Here's how the part is built. I have some questions about the finished solid (model axes, mm). Give positions to 0.01 mm unless a question says otherwise; leave off trailing zeros. Order: outer loops, then holes, each group sorted by start corner. A loop starts at its lowest first (then second) coordinate and runs counter-clockwise, first axis right, second up.
from build123d import *

# Parameters (mm, degrees)
BOSS_EXTRUDE4_DEPTH = 200
SKETCH3_R           = 2
CUT_EXTRUDE1_DEPTH  = 200
SKETCH3_3_R         = 3
SKETCH3_3_R_2       = 2
CUT_EXTRUDE2_DEPTH  = 2.5
SKETCH4_W           = 36.815771896
SKETCH4_H           = 9
CUT_EXTRUDE3_DEPTH  = 10


with BuildPart() as part:
    # Sketch1 → Boss-Extrude4 (new body)
    with BuildSketch(Plane.XY):
        with BuildLine():
            Line((10.168613541, -5.014716436), (10.168390302, 3.235283561))
            Line((10.168390302, 3.235283561), (9.793380155, 3.610273413))
            Line((9.793380155, 3.610273413), (7.005880156, 3.610197985))
            Line((7.005880156, 3.610197985), (6.630890303, 3.235187838))
            Line((6.630890303, 3.235187838), (6.630908906, 2.547687839))
            ThreePointArc((6.630908906, 2.547687839), (6.508267883, 2.251583555), (6.212170237, 2.128926508))
            ThreePointArc((6.212170237, 2.128926508), (5.916065954, 2.251567531), (5.793408907, 2.547665177))
            Line((5.793408907, 2.547665177), (5.793390303, 3.235165176))
            Line((5.793390303, 3.235165176), (5.418380156, 3.610155029))
            Line((5.418380156, 3.610155029), (4.793380156, 3.610138117))
            Line((4.793380156, 3.610138117), (4.168397069, 2.985121205))
            Line((4.168397069, 2.985121205), (4.168606778, -4.764878792))
            Line((4.168606778, -4.764878792), (4.79362369, -5.38986188))
            Line((4.79362369, -5.38986188), (5.41862369, -5.389844968))
            Line((5.41862369, -5.389844968), (5.793613542, -5.014834821))
            Line((5.793613542, -5.014834821), (5.793594939, -4.327334821))
            ThreePointArc((5.793594939, -4.327334821), (6.212333608, -3.90857349), (6.631094939, -4.327312159))
            Line((6.631094939, -4.327312159), (6.631113542, -5.014812159))
            Line((6.631113542, -5.014812159), (7.006123689, -5.389802011))
            Line((7.006123689, -5.389802011), (9.793623688, -5.389726583))
            Line((9.793623688, -5.389726583), (10.168613541, -5.014716436))
        make_face()
    extrude(amount=BOSS_EXTRUDE4_DEPTH)

    # Sketch3 → Cut-Extrude1 (cut)
    with BuildSketch(Plane(origin=(4.168477841, 0.000112796, 0), x_dir=(0, 0, 1), z_dir=(-0.999999999633898, -2.7059269393071615e-05, 0))):
        with Locations(Location((9, -0.88999159, 0), (0, 0, 270))):
            Circle(SKETCH3_R)
        with Locations(Location((29, -0.88999159, 0), (0, 0, 270))):
            Circle(SKETCH3_R)
        with Locations(Location((49, -0.88999159, 0), (0, 0, 270))):
            Circle(SKETCH3_R)
        with Locations(Location((69, -0.88999159, 0), (0, 0, 270))):
            Circle(SKETCH3_R)
        with Locations(Location((89, -0.88999159, 0), (0, 0, 270))):
            Circle(SKETCH3_R)
        with Locations(Location((109, -0.88999159, 0), (0, 0, 270))):
            Circle(SKETCH3_R)
        with Locations(Location((129, -0.88999159, 0), (0, 0, 270))):
            Circle(SKETCH3_R)
        with Locations(Location((149, -0.88999159, 0), (0, 0, 270))):
            Circle(SKETCH3_R)
        with Locations(Location((169, -0.88999159, 0), (0, 0, 270))):
            Circle(SKETCH3_R)
        with Locations(Location((189, -0.88999159, 0), (0, 0, 270))):
            Circle(SKETCH3_R)
    extrude(amount=-CUT_EXTRUDE1_DEPTH, mode=Mode.SUBTRACT)

    # Sketch3_3 → Cut-Extrude2 (cut)
    # profile 1 of 10: a face of its own
    with BuildSketch(Plane(origin=(4.168477841, 0.000112796, 0), x_dir=(0, 0, 1), z_dir=(-0.999999999633898, -2.7059269393071615e-05, 0))):
        with Locations(Location((9, -0.88999159, 0), (0, 0, 270))):
            Circle(SKETCH3_3_R)
        with Locations(Location((9, -0.88999159, 0), (0, 0, 270))):
            Circle(SKETCH3_3_R_2, mode=Mode.SUBTRACT)
    # profile 2 of 10: a face of its own
    with BuildSketch(Plane(origin=(4.168477841, 0.000112796, 0), x_dir=(0, 0, 1), z_dir=(-0.999999999633898, -2.7059269393071615e-05, 0))):
        with Locations(Location((29, -0.88999159, 0), (0, 0, 270))):
            Circle(SKETCH3_3_R)
        with Locations(Location((29, -0.88999159, 0), (0, 0, 270))):
            Circle(SKETCH3_3_R_2, mode=Mode.SUBTRACT)
    # profile 3 of 10: a face of its own
    with BuildSketch(Plane(origin=(4.168477841, 0.000112796, 0), x_dir=(0, 0, 1), z_dir=(-0.999999999633898, -2.7059269393071615e-05, 0))):
        with Locations(Location((49, -0.88999159, 0), (0, 0, 270))):
            Circle(SKETCH3_3_R)
        with Locations(Location((49, -0.88999159, 0), (0, 0, 270))):
            Circle(SKETCH3_3_R_2, mode=Mode.SUBTRACT)
    # profile 4 of 10: a face of its own
    with BuildSketch(Plane(origin=(4.168477841, 0.000112796, 0), x_dir=(0, 0, 1), z_dir=(-0.999999999633898, -2.7059269393071615e-05, 0))):
        with Locations(Location((69, -0.88999159, 0), (0, 0, 270))):
            Circle(SKETCH3_3_R)
        with Locations(Location((69, -0.88999159, 0), (0, 0, 270))):
            Circle(SKETCH3_3_R_2, mode=Mode.SUBTRACT)
    # profile 5 of 10: a face of its own
    with BuildSketch(Plane(origin=(4.168477841, 0.000112796, 0), x_dir=(0, 0, 1), z_dir=(-0.999999999633898, -2.7059269393071615e-05, 0))):
        with Locations(Location((89, -0.88999159, 0), (0, 0, 270))):
            Circle(SKETCH3_3_R)
        with Locations(Location((89, -0.88999159, 0), (0, 0, 270))):
            Circle(SKETCH3_3_R_2, mode=Mode.SUBTRACT)
    # profile 6 of 10: a face of its own
    with BuildSketch(Plane(origin=(4.168477841, 0.000112796, 0), x_dir=(0, 0, 1), z_dir=(-0.999999999633898, -2.7059269393071615e-05, 0))):
        with Locations(Location((109, -0.88999159, 0), (0, 0, 270))):
            Circle(SKETCH3_3_R)
        with Locations(Location((109, -0.88999159, 0), (0, 0, 270))):
            Circle(SKETCH3_3_R_2, mode=Mode.SUBTRACT)
    # profile 7 of 10: a face of its own
    with BuildSketch(Plane(origin=(4.168477841, 0.000112796, 0), x_dir=(0, 0, 1), z_dir=(-0.999999999633898, -2.7059269393071615e-05, 0))):
        with Locations(Location((129, -0.88999159, 0), (0, 0, 270))):
            Circle(SKETCH3_3_R)
        with Locations(Location((129, -0.88999159, 0), (0, 0, 270))):
            Circle(SKETCH3_3_R_2, mode=Mode.SUBTRACT)
    # profile 8 of 10: a face of its own
    with BuildSketch(Plane(origin=(4.168477841, 0.000112796, 0), x_dir=(0, 0, 1), z_dir=(-0.999999999633898, -2.7059269393071615e-05, 0))):
        with Locations(Location((149, -0.88999159, 0), (0, 0, 270))):
            Circle(SKETCH3_3_R)
        with Locations(Location((149, -0.88999159, 0), (0, 0, 270))):
            Circle(SKETCH3_3_R_2, mode=Mode.SUBTRACT)
    # profile 9 of 10: a face of its own
    with BuildSketch(Plane(origin=(4.168477841, 0.000112796, 0), x_dir=(0, 0, 1), z_dir=(-0.999999999633898, -2.7059269393071615e-05, 0))):
        with Locations(Location((169, -0.88999159, 0), (0, 0, 270))):
            Circle(SKETCH3_3_R)
        with Locations(Location((169, -0.88999159, 0), (0, 0, 270))):
            Circle(SKETCH3_3_R_2, mode=Mode.SUBTRACT)
    # profile 10 of 10: a face of its own
    with BuildSketch(Plane(origin=(4.168477841, 0.000112796, 0), x_dir=(0, 0, 1), z_dir=(-0.999999999633898, -2.7059269393071615e-05, 0))):
        with Locations(Location((189, -0.88999159, 0), (0, 0, 270))):
            Circle(SKETCH3_3_R)
        with Locations(Location((189, -0.88999159, 0), (0, 0, 270))):
            Circle(SKETCH3_3_R_2, mode=Mode.SUBTRACT)
    extrude(amount=-CUT_EXTRUDE2_DEPTH, mode=Mode.SUBTRACT)

    # Sketch4 → Cut-Extrude3 (cut)
    with BuildSketch(Plane(origin=(10.168477839, 0.000275152, 0), x_dir=(0, 0, -1), z_dir=(0.999999999633898, 2.7059269386201862e-05, 0))):
        with Locations((-181.592114052, -0.88999159)):
            Rectangle(SKETCH4_W, SKETCH4_H)
    extrude(amount=-CUT_EXTRUDE3_DEPTH, mode=Mode.SUBTRACT)


solid = part.part
Q1. I'm going to push a flat-ended pin straight in: P1, Ø3, axis at y = -0.89, z = 69, coming from the -X side. Where does the tip first touch, or does it pass through?
Filled sheet:
P1: passes through
Q2. I need wall thicknesses on L1, parallel to X at y = 2.5, z = 9; L2, parallel to Y at x = 5.45, z = 129; L3, parallel to X at y = -4, z = 105. Which ranges of each line are inside material? Lowest first, please.
Filled sheet:
L1: x = 4.17 to 5.8, 6.63 to 10.17
L2: y = -5.36 to -3.89, 2.11 to 3.58
L3: x = 4.17 to 5.95, 6.47 to 10.17
Q3. If we section it at B-B on x = 8.25: Give the number of separate pieces and of enclosed holes in the cut face, plus the area to 3 significant figures.
Filled sheet:
separate pieces: 1
enclosed holes: 8
area: 1,370 mm2
Q4. If we section it at A-A on z = 69: List the corners of the cut face in (x, y) for me, plus the area to 3 significant figures.
Filled sheet:
outline: (4.17, -4.76) - (4.79, -5.39) - (5.42, -5.39) - (5.79, -5.01) - (5.79, -4.33) arc R0.42 cw to (6.63, -4.33) - (6.63, -5.01) - (7.01, -5.39) - (9.79, -5.39) - (10.17, -5.01) - (10.17, -2.89) - (6.67, -2.89) - (6.67, -3.89) - (4.17, -3.89) - close; (4.17, 2.11) - (6.67, 2.11) - (6.67, 1.11) - (10.17, 1.11) - (10.17, 3.24) - (9.79, 3.61) - (7.01, 3.61) - (6.63, 3.24) - (6.63, 2.55) arc R0.42 cw to (5.79, 2.55) - (5.79, 3.24) - (5.42, 3.61) - (4.79, 3.61) - (4.17, 2.99) - close
area: 21.9 mm2
